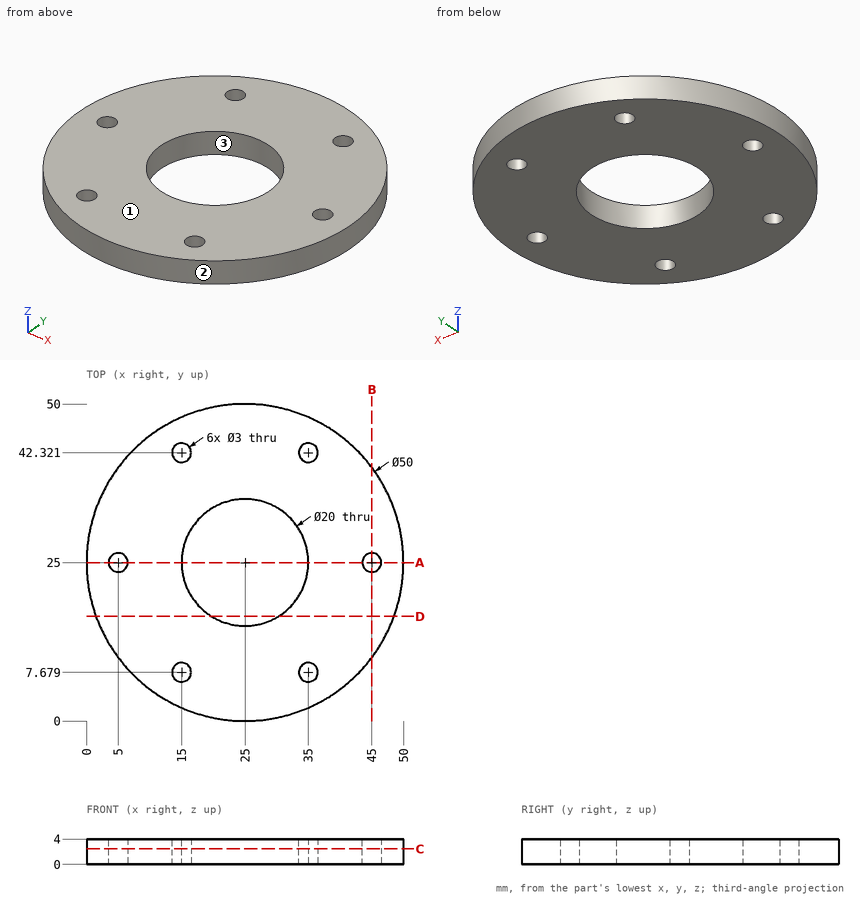
Design review of the part shown in the three views and the two pictorial views. Dimensions are in mm from the part's minimum x, y and z. Give positions to 0.01 mm unless a question says otherwise; leave off trailing zeros. Loops run counter-clockwise (first coordinate to the right, second up) from the corner with the lowest first, then second, coordinate; pieces in that order, holes last. Notation, with made-up numbers: M -14,12.25 L 30,12.25 A27 ccw 30,50.25 Z; hole C 22.25,74.25 d1. An arc over 180 degrees is marked long. Answer as a JSON object with one key per item and string values. Group by question number.
Q1. Mouldability with a two-part tool opening along X and no side actions: class the marked faces 1, 2 and 3 as +X half, -X half, draft (parallel to the pull), parting line (faces both ways), or undercut.
Q2. Add section D-D on y = 16.5. Give the boundary of the cut face in (x, z), and give its area (3 significant figures).
Q3. Add section A-A on y = 25. Give the boundary of the cut face in (x, z).
Q4. Add section C-C on z = 2.45. Give the boundary of the cut face in (x, y).
Q5. Insertion check: P1, Ø2.5, axis at x = 45, y = 25, coming from the -Z side; P2, Ø1.5, axis at y = 5.5, z = 2.5, coming from the +X side (1 decimal). Each pin has a flat end and moves straight along its axis. Give the tip position at first contact, or say it passes through.
Q6. Add section B-B on x = 45. Give the boundary of the cut face in (y, z), and give its area (3 significant figures).
Q7. For probe 1 along X at (y, z) = (23, 3.45); probe 2 along X at (y, z) = (9, 3.25) (1 decimal); probe 3 along Y at (x, z) = (45, 1.45), list the stretches that pass through material, from the lowest coordinate up. Write a range as [from, to].
Checked values:
{
 "1": {"face 1": "draft", "face 2": "parting line", "face 3": "undercut"},
 "2": {"outline": "M 1.49,0 L 19.73,0 L 19.73,4 L 1.49,4 Z; M 30.27,0 L 48.51,0 L 48.51,4 L 30.27,4 Z", "area": "146 mm²"},
 "3": {"outline": "M 0,0 L 3.5,0 L 3.5,4 L 0,4 Z; M 6.5,0 L 15,0 L 15,4 L 6.5,4 Z; M 35,0 L 43.5,0 L 43.5,4 L 35,4 Z; M 46.5,0 L 50,0 L 50,4 L 46.5,4 Z"},
 "4": {"outline": "C 25,25 d50; hole C 5,25 d3; hole C 15,7.68 d3; hole C 15,42.32 d3; hole C 25,25 d20; hole C 35,7.68 d3; hole C 35,42.32 d3; hole C 45,25 d3"},
 "5": {"P1": "through", "P2": "x = 41.5"},
 "6": {"outline": "M 10,0 L 23.5,0 L 23.5,4 L 10,4 Z; M 26.5,0 L 40,0 L 40,4 L 26.5,4 Z", "area": "108 mm²"},
 "7": {"probe 1": "[0.08, 15.2], [34.8, 49.92]", "probe 2": "[5.8, 14.3], [15.7, 34.3], [35.7, 44.2]", "probe 3": "[10, 23.5], [26.5, 40]"}
}
